Here's the drawing with two shaded views (mm, measured from the low corner). I have some questions. A direction names the side the tool comes from. Round coordinates to 2 decimals unless told otherwise and drop trailing zeros. Loops run counter-clockwise (first coordinate to the right, second up) from the corner with the lowest first, then second, coordinate; pieces in that order, holes last.
(1) Will these pins go through, and if not, where does the flat tip stop? pin 1 Ø5 at (x, y) = (10, 10) entering from +Z; pin 2 Ø1.5 at (y, z) = (3, 2.5) entering from +X; pin 3 Ø5 at (x, y) = (10, 10) entering from -Z; pin 4 Ø2 at (x, z) = (15, 2.5) entering from -Y.
(2) Which directions (+Z, -Z, +X, -X, +Y, -Y) give clear straight access to the entire face, cutting with the end or side of a thin tool? Please do the marked faces 4 and 5.
(3) I want a section at A-A on x = 10. Write out the boundary of the cut face in (y, z), plus the area to 3 significant figures.
(4) I want a section at C-C on z = 5. Write out the boundary of the cut face in (x, y).
(5) Thinking about a two-plate mould opening in Y: for the marked faces 1, 2 and 3, which applies, released by +Y, released by -Y, zero draft, split by the parting line, or undercut?
(6) If I drill on line 1 along Y through (x, z) = (10, 4.8); line 2 along Z through (x, y) = (7, 4), over which ranges is the centre line in solid material (lowest first)?
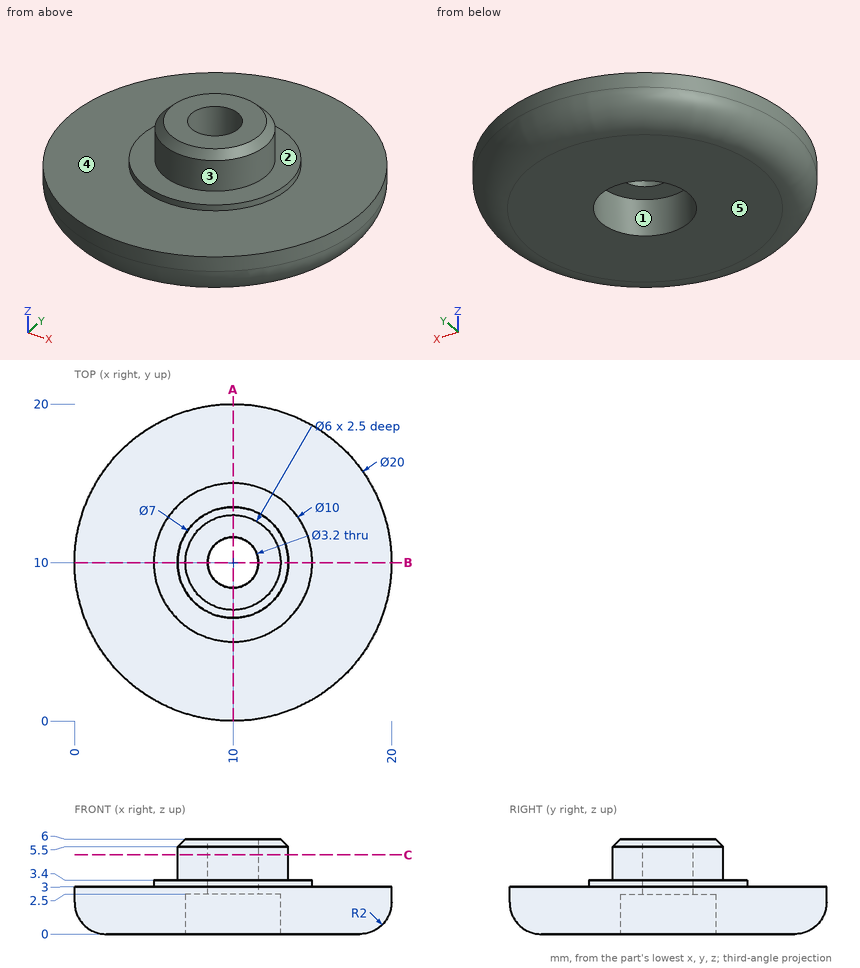
Filled sheet:
1. pin 1: stops at z = 6
1. pin 2: stops at x = 17.81
1. pin 3: stops at z = 2.5
1. pin 4: stops at y = 0.83
2. face 4: +Z
2. face 5: -Z, +X, -X, +Y, -Y
3. outline: (0, 2) arc R2 ccw to (2, 0) - (7, 0) - (7, 2.5) - (8.4, 2.5) - (8.4, 6) - (7, 6) - (6.5, 5.5) - (6.5, 3.4) - (5, 3.4) - (5, 3) - (0, 3) - close; (11.6, 2.5) - (13, 2.5) - (13, 0) - (18, 0) arc R2 ccw to (20, 2) - (20, 3) - (15, 3) - (15, 3.4) - (13.5, 3.4) - (13.5, 5.5) - (13, 6) - (11.6, 6) - close
3. area: 54.0 mm2
4. outline: circle Ø7 at (10, 10); hole circle Ø3.2 at (10, 10)
5. face 1: undercut
5. face 2: zero draft
5. face 3: split by the parting line
6. line 1: y = 6.5 to 8.4, 11.6 to 13.5
6. line 2: z = 0 to 3
